from build123d import *

# Parameters (mm, degrees)
F1_DEPTH = 25
F2_R     = 8
F3_W     = 23.684212938
F3_H     = 3.5125516355
F4_DEPTH = 25
F5_W     = 5.4730284959
F5_H     = 39.9671059567
F6_DEPTH = 25
F7_R     = 3.8177779447
F8_DEPTH = 25


with BuildPart() as f1:
    # F0 (on Front) → F1 (new body)
    with BuildSketch(Plane.XZ):
        Polygon((0, -10.2138156071), (0, 17.9111845791), (-19.6875017136, 17.9111845791), (-19.6875017136, 3.848684486), (-19.6875017136, 0), (-19.6875017136, -10.2138156071), align=None)
        Polygon((-19.6875017136, 0), (-19.6875017136, 3.848684486), (-43.3717146516, 3.848684486), (-43.3717146516, 41.8914481997), (-46.3322401047, 41.8914481997), (-46.3322401047, 0), align=None)
    extrude(amount=F1_DEPTH)

    # F2
    f2_edges = [f1.edges().sort_by_distance(p)[0] for p in [
        (-9.843751, 0, 17.911185),
        (-9.843751, 0, -10.213816),
        (-9.843751, -25, -10.213816),
        (-9.843751, -25, 17.911185),
    ]]
    fillet(f2_edges, radius=F2_R)

    # F3 (on face) → F4 (cut)
    with BuildSketch(Plane.XY.offset(3.848684486)):
        with Locations((-31.5296081826, -23.2437241822)):
            Rectangle(F3_W, F3_H)
        Polygon((-43.3717146516, -4.7452212311), (-19.6875017136, -4.2484635487), (-19.6875017136, 0), (-20.5312147737, 0), (-43.3717146516, 0), align=None)
    extrude(amount=-F4_DEPTH, mode=Mode.SUBTRACT)

    # F5 (on face) → F6 (cut)
    with BuildSketch(Plane.YZ.offset(-43.3717146516)):
        with Locations((-22.263485752, 21.9078952214)):
            Rectangle(F5_W, F5_H)
        Polygon((0, 41.8914481997), (-4.7452212311, 41.8914481997), (-3.9370520972, 0), (0, 0), (0, 40.7377965748), align=None)
    extrude(amount=-F6_DEPTH, mode=Mode.SUBTRACT)

    # F7 (on face) → F8 (cut)
    with BuildSketch(Plane(origin=(-46.3322401047, 0, 0), x_dir=(0, -1, 0), z_dir=(-1, 0, 0))):
        with Locations((9.3853315338, 35.6243662536)):
            Circle(F7_R)
    extrude(amount=-F8_DEPTH, mode=Mode.SUBTRACT)

    # F9: F1 across plane


with BuildPart() as f1_1:
    add(f1.part)
    add(f1.part.mirror(Plane.YZ))


solid = f1_1.part
Geometry check sheet. Reference: the model listing, model coordinates, mm. A direction names the side the tool comes from. Give positions to 0.01 mm unless a question says otherwise; leave off trailing zeros. Write each loop counter-clockwise with the first axis right and the second up, starting at its lowest first coordinate (ties: lowest second). Pieces come first, ordered by that corner, then holes. Notation, with made-up numbers: M 41.5,24 L 87.5,24 A24 cw 87.5,55 Z; hole C 31.5,4.25 d2. An arc over 180 degrees is marked long. Answer as CSV lines item,"result". Start each with the question number.
Q1. Section check A-A, the plane z = 20. Record the cut outline in (x, y), then the cut area to 3 significant figures.
Q2. Section check C-C, the plane z = 7.5. Record the cut outline in (x, y), then the cut area to 3 significant figures.
Q3. Material ranges on L1, parallel to X at y = -18.5, z = 9.5; L2, parallel to X at y = -16.25, z = 30.5; L3, parallel to Z at x = 33, y = -7, recorded low to high.
Q4. Section check D-D, the plane y = -2.5. Record the cut outline in (x, z), then the cut area to 3 significant figures.
Q5. Tool access check on faces 1 (the face through (33, -14, 0)), 2 (the face through (31, -13, 3.849)), 3 (the face through (32, -21.487, 2)), 4 (the face through (-0.276, -22.594, -7.933)), 5 (the face through (-33, -14, 0)). Record the directions out of +Z, -Z, +X, -X, +Y, -Y that give a thin tool (end or side, any length) a straight path to the whole face; none if there is none.
Q6. Go/stop test with flat-tipped pins: pin 1 (3 mm diameter, centred on x = -35.5, z = 3, fed in from -Y); pin 2 (1.5 mm diameter, centred on y = -21, z = 3, fed in from +X); pin 3 (10.5 mm diameter, centred on x = 37.5, y = -13.5, fed in from -Z); pin 4 (6 mm diameter, centred on y = -9.39, z = 35.62, fed in from +X). Record where each tip stops, or that it passes through.
Q7. Release check for a two-part mould opening along Y. For faces 6 (the face through (-45, -19.527, 22)), 7 (the face through (44.87, -8.89, 39.41)), 8 (the face through (19.688, -12, 4)), 9 (the face through (0, 0, 4)) record: pulls with the +Y half, pulls with the -Y half, needs draft (parallel to the pull), parting line crosses it, or undercut.
Q8. Section check B-B, the plane x = -18.5. Record the cut outline in (y, z).
Geometry says:
1,outline,"M -46.33,-19.53 L -43.37,-19.53 L -43.37,-4.32 L -46.33,-4.32 Z; M 43.37,-19.53 L 46.33,-19.53 L 46.33,-4.32 L 43.37,-4.32 Z"
1,area,"90.0 mm^2"
2,outline,"M -46.33,-19.53 L -43.37,-19.53 L -43.37,-4.08 L -46.33,-4.08 Z; M -19.69,-25 L 19.69,-25 L 19.69,0 L -19.69,0 Z; M 43.37,-19.53 L 46.33,-19.53 L 46.33,-4.08 L 43.37,-4.08 Z"
2,area,"1,080 mm^2"
3,L1,"-46.33 to -43.37, -19.69 to 19.69, 43.37 to 46.33"
3,L2,"-46.33 to -43.37, 43.37 to 46.33"
3,L3,"0 to 3.85"
4,outline,"M -19.69,-8.02 L 19.69,-8.02 L 19.69,15.72 L -19.69,15.72 Z"
4,area,"935 mm^2"
5,face 1,"-Z, +X, +Y, -Y"
5,face 2,"+Z, +Y, -Y"
5,face 3,"+Z, -Z, -Y"
5,face 4,"-Z, +X, -X, -Y"
5,face 5,"-Z, -X, +Y, -Y"
6,pin 1,"y = -21.49"
6,pin 2,"x = 43.37"
6,pin 3,"z = 0"
6,pin 4,"through"
7,face 6,"pulls with the -Y half"
7,face 7,"undercut"
7,face 8,"needs draft"
7,face 9,"pulls with the +Y half"
8,outline,"M -25,-2.21 A8 ccw -17,-10.21 L -8,-10.21 A8 ccw 0,-2.21 L 0,9.91 A8 ccw -8,17.91 L -17,17.91 A8 ccw -25,9.91 Z"
